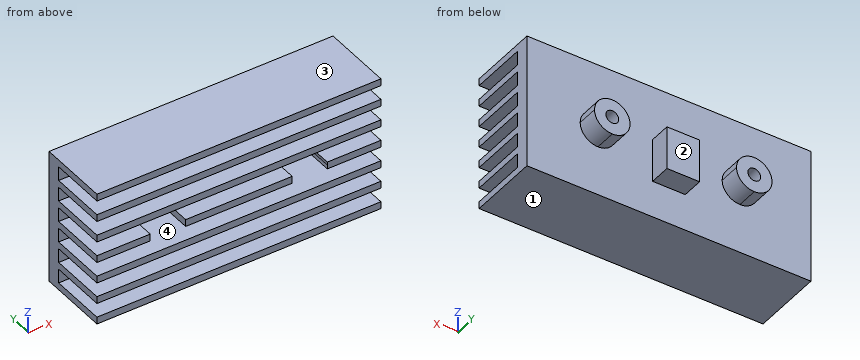
from build123d import *

# Parameters (mm, degrees)
F0_W     = 40
F0_H     = 19
F1_DEPTH = 10
F2_W     = 40
F2_H     = 2
F4_DEPTH = 8
F5_R     = 0.9
F5_W     = 4.6
F5_H     = 6.1
F7_DEPTH = 5
F8_DEPTH = 8.001
F9_DEPTH = 5.001


# Not quite as in the source:
# - a feature names something its author has since deleted; it is built from what else it names


with BuildPart() as f1:
    # F0 (on Front) → F1 (new body)
    with BuildSketch(Plane.XZ):
        Rectangle(F0_W, F0_H)
    extrude(amount=F1_DEPTH)

    # F2 (on face) → F4 (cut, through all)
    with BuildSketch(Plane.XZ.offset(10)):
        with Locations((0, 7.5)):
            Rectangle(F2_W, F2_H)
        with Locations((0, 4.5)):
            Rectangle(F2_W, F2_H)
        with Locations((0, 1.5)):
            Rectangle(F2_W, F2_H)
        with Locations((0, -1.5)):
            Rectangle(F2_W, F2_H)
        with Locations((0, -4.5)):
            Rectangle(F2_W, F2_H)
        with Locations((0, -7.5)):
            Rectangle(F2_W, F2_H)
    extrude(amount=-F4_DEPTH, mode=Mode.SUBTRACT)

    # F5 (on offset) → F7 (join, through all)
    with BuildSketch(Plane.XZ.offset(2)):
        with BuildLine():
            ThreePointArc((10, 2.5), (8.232233047, 1.767766953), (7.5, 0))
            ThreePointArc((7.5, 0), (8.232233047, -1.767766953), (10, -2.5))
            ThreePointArc((10, -2.5), (11.767766953, -1.767766953), (12.5, 0))
            ThreePointArc((12.5, 0), (11.767766953, 1.767766953), (10, 2.5))
        make_face()
        with Locations((10, 0)):
            Circle(F5_R, mode=Mode.SUBTRACT)
        with BuildLine():
            ThreePointArc((-10, -2.5), (-8.232233047, -1.767766953), (-7.5, 0))
            ThreePointArc((-7.5, 0), (-8.232233047, 1.767766953), (-10, 2.5))
            ThreePointArc((-10, 2.5), (-11.767766953, 1.767766953), (-12.5, 0))
            ThreePointArc((-12.5, 0), (-11.767766953, -1.767766953), (-10, -2.5))
        make_face()
        with Locations((-10, 0)):
            Circle(F5_R, mode=Mode.SUBTRACT)
        with Locations((0, -1.25)):
            Rectangle(F5_W, F5_H)
    extrude(amount=-F7_DEPTH)

    # F5 (on offset) → F8 (cut, through all)
    with BuildSketch(Plane.XZ.offset(2)):
        with BuildLine():
            ThreePointArc((-10, 2.5), (-8.232233047, 1.767766953), (-7.5, 0))
            Line((-7.5, 0), (-7.5, 2.5))
            Line((-7.5, 2.5), (-10, 2.5))
        make_face()
        with BuildLine():
            ThreePointArc((-12.5, 0), (-11.767766953, 1.767766953), (-10, 2.5))
            Line((-10, 2.5), (-12.5, 2.5))
            Line((-12.5, 2.5), (-12.5, 0))
        make_face()
        with BuildLine():
            Line((-12.5, -2.5), (-10, -2.5))
            ThreePointArc((-10, -2.5), (-11.767766953, -1.767766953), (-12.5, 0))
            Line((-12.5, 0), (-12.5, -2.5))
        make_face()
        with BuildLine():
            Line((-7.5, -2.5), (-7.5, 0))
            ThreePointArc((-7.5, 0), (-8.232233047, -1.767766953), (-10, -2.5))
            Line((-10, -2.5), (-7.5, -2.5))
        make_face()
        with BuildLine():
            ThreePointArc((-10, -2.5), (-8.232233047, -1.767766953), (-7.5, 0))
            ThreePointArc((-7.5, 0), (-8.232233047, 1.767766953), (-10, 2.5))
            ThreePointArc((-10, 2.5), (-11.767766953, 1.767766953), (-12.5, 0))
            ThreePointArc((-12.5, 0), (-11.767766953, -1.767766953), (-10, -2.5))
        make_face()
        with Locations((-10, 0)):
            Circle(F5_R, mode=Mode.SUBTRACT)
        with Locations((-10, 0)):
            Circle(F5_R)
        with BuildLine():
            Line((10, 2.5), (7.5, 2.5))
            Line((7.5, 2.5), (7.5, 0))
            ThreePointArc((7.5, 0), (8.232233047, 1.767766953), (10, 2.5))
        make_face()
        with BuildLine():
            ThreePointArc((10, -2.5), (8.232233047, -1.767766953), (7.5, 0))
            Line((7.5, 0), (7.5, -2.5))
            Line((7.5, -2.5), (10, -2.5))
        make_face()
        with BuildLine():
            ThreePointArc((10, 2.5), (8.232233047, 1.767766953), (7.5, 0))
            ThreePointArc((7.5, 0), (8.232233047, -1.767766953), (10, -2.5))
            ThreePointArc((10, -2.5), (11.767766953, -1.767766953), (12.5, 0))
            ThreePointArc((12.5, 0), (11.767766953, 1.767766953), (10, 2.5))
        make_face()
        with Locations((10, 0)):
            Circle(F5_R, mode=Mode.SUBTRACT)
        with Locations((10, 0)):
            Circle(F5_R)
    extrude(amount=F8_DEPTH, mode=Mode.SUBTRACT)

    # F5 (on offset) → F9 (cut, through all)
    with BuildSketch(Plane.XZ.offset(2)):
        with Locations((10, 0)):
            Circle(F5_R)
        with Locations((-10, 0)):
            Circle(F5_R)
    extrude(amount=-F9_DEPTH, mode=Mode.SUBTRACT)


solid = f1.part
Here's how the part is built. I have some questions about the finished solid (model axes, mm). Face numbers are marked on the shaded views. Round coordinates to 2 decimals unless told otherwise and drop trailing zeros. Write each loop counter-clockwise with the first axis right and the second up, starting at its lowest first coordinate (ties: lowest second). Pieces come first, ordered by that corner, then holes.
1. I need wall thicknesses on L1, parallel to Z at x = 8.5, y = -2.75; L2, parallel to Z at x = 10, y = 1.4; L3, parallel to Z at x = 10, y = -0.5. Which ranges of each line are inside material? Lowest first, please.
2. Will this pin go through, and if not, where does the flat tip stop? pin 1 Ø1 at (x, z) = (-1, 5) entering from +Y.
3. Suppose I cut it at B-B (y = -4.25). State how many separate pieces and enclosed holes the cut face has, and give its area (3 significant figures).
4. Suppose I cut it at C-C (z = 3). List the corners of the cut face in (x, y) for me.
5. If we mould it in two halves opening along Z, with no side actions, what happens to the marked faces 1, 2, 3 and 4? For each: released by +Z, released by -Z, zero draft, split by the parting line, or undercut.
Answer sheet:
1. L1: z = -9.5 to -8.5, -6.5 to -5.5, -3.5 to -2.5, 2.5 to 3.5, 5.5 to 6.5, 8.5 to 9.5
1. L2: z = -2.5 to -0.9, 0.9 to 2.5
1. L3: z = -9.5 to -0.9, 0.9 to 9.5
2. pin 1: stops at y = 0
3. separate pieces: 9
3. enclosed holes: 0
3. area: 270 mm2
4. outline: (-20, -10) - (20, -10) - (20, 0) - (-20, 0) - close
5. face 1: released by -Z
5. face 2: zero draft
5. face 3: released by +Z
5. face 4: undercut
